from build123d import *

# Parameters (mm, degrees)
SKETCH1_R           = 15
BOSS_EXTRUDE1_DEPTH = 3


with BuildPart() as part:
    # Sketch1 → Boss-Extrude1 (new body)
    with BuildSketch(Plane(origin=(0, 0, 0), x_dir=(1, 0, 0), z_dir=(0, 1, 0))):
        with Locations(Location((0, 0, 0), (0, 0, 270))):
            Circle(SKETCH1_R)
        with BuildLine():
            Line((-1.118033989, 1), (1.118033989, 1))
            ThreePointArc((1.118033989, 1), (0, -1.5), (-1.118033989, 1))
        make_face(mode=Mode.SUBTRACT)
        with BuildLine():
            Line((-12.557368355, -7.25), (-10.392304845, -6))
            ThreePointArc((-10.392304845, -6), (-9.192533317, -7.713451316), (-7.713451316, -9.192533317))
            Line((-7.713451316, -9.192533317), (-9.32042034, -11.107644425))
            ThreePointArc((-9.32042034, -11.107644425), (-11.107644425, -9.32042034), (-12.557368355, -7.25))
        make_face(mode=Mode.SUBTRACT)
        with BuildLine():
            Line((-4.959292078, -13.625543001), (-4.10424172, -11.276311449))
            ThreePointArc((-4.10424172, -11.276311449), (-2.083778132, -11.817693036), (0, -12))
            Line((0, -12), (0, -14.5))
            ThreePointArc((0, -14.5), (-2.517898576, -14.279712419), (-4.959292078, -13.625543001))
        make_face(mode=Mode.SUBTRACT)
        with BuildLine():
            Line((4.959292078, -13.625543001), (4.10424172, -11.276311449))
            ThreePointArc((4.10424172, -11.276311449), (6, -10.392304845), (7.713451316, -9.192533317))
            Line((7.713451316, -9.192533317), (9.32042034, -11.107644425))
            ThreePointArc((9.32042034, -11.107644425), (7.25, -12.557368355), (4.959292078, -13.625543001))
        make_face(mode=Mode.SUBTRACT)
        with BuildLine():
            Line((12.557368355, -7.25), (10.392304845, -6))
            ThreePointArc((10.392304845, -6), (11.276311449, -4.10424172), (11.817693036, -2.083778132))
            Line((11.817693036, -2.083778132), (14.279712419, -2.517898576))
            ThreePointArc((14.279712419, -2.517898576), (13.625543001, -4.959292078), (12.557368355, -7.25))
        make_face(mode=Mode.SUBTRACT)
        with BuildLine():
            Line((-14.279712419, 2.517898576), (-11.817693036, 2.083778132))
            ThreePointArc((-11.817693036, 2.083778132), (-12, 0), (-11.817693036, -2.083778132))
            Line((-11.817693036, -2.083778132), (-14.279712419, -2.517898576))
            ThreePointArc((-14.279712419, -2.517898576), (-14.5, 0), (-14.279712419, 2.517898576))
        make_face(mode=Mode.SUBTRACT)
        with BuildLine():
            Line((-9.32042034, 11.107644425), (-7.713451316, 9.192533317))
            ThreePointArc((-7.713451316, 9.192533317), (-9.192533317, 7.713451316), (-10.392304845, 6))
            Line((-10.392304845, 6), (-12.557368355, 7.25))
            ThreePointArc((-12.557368355, 7.25), (-11.107644425, 9.32042034), (-9.32042034, 11.107644425))
        make_face(mode=Mode.SUBTRACT)
        with BuildLine():
            Line((-4.10424172, 11.276311449), (-4.959292078, 13.625543001))
            ThreePointArc((-4.959292078, 13.625543001), (-2.517898576, 14.279712419), (0, 14.5))
            Line((0, 14.5), (0, 12))
            ThreePointArc((0, 12), (-2.083778132, 11.817693036), (-4.10424172, 11.276311449))
        make_face(mode=Mode.SUBTRACT)
        with BuildLine():
            ThreePointArc((11.817693036, 2.083778132), (11.276311449, 4.10424172), (10.392304845, 6))
            Line((10.392304845, 6), (12.557368355, 7.25))
            ThreePointArc((12.557368355, 7.25), (13.625543001, 4.959292078), (14.279712419, 2.517898576))
            Line((14.279712419, 2.517898576), (11.817693036, 2.083778132))
        make_face(mode=Mode.SUBTRACT)
        with BuildLine():
            Line((9.32042034, 11.107644425), (7.713451316, 9.192533317))
            ThreePointArc((7.713451316, 9.192533317), (6, 10.392304845), (4.10424172, 11.276311449))
            Line((4.10424172, 11.276311449), (4.959292078, 13.625543001))
            ThreePointArc((4.959292078, 13.625543001), (7.25, 12.557368355), (9.32042034, 11.107644425))
        make_face(mode=Mode.SUBTRACT)
    extrude(amount=BOSS_EXTRUDE1_DEPTH)


solid = part.part
The listing builds one solid part. Answer for the finished solid, in the listing's coordinates (mm). Coordinates: 2 decimals unless noted, no trailing zeros. Write each loop counter-clockwise with the first axis right and the second up, starting at its lowest first coordinate (ties: lowest second). Pieces come first, ordered by that corner, then holes. Notation, with made-up numbers: M -35.5,28 L 21.5,28 A22 cw 21.5,61 Z; hole C 12,-31.75 d7. An arc over 180 degrees is marked long. Put each result on its own line as item: value. Start each with the question number.
1. Consider line 1 (X direction, y = 1, z = 6.25); line 2 (Z direction, x = 5, y = 0.45); line 3 (Z direction, x = -2.75, y = 0.45). Determine where each line is inside the solid, lowest interval first. Write a range as from..to.
2. Flat-ended cylindrical pins translate along their axes: P1, Ø4, axis at x = -12, z = -7.5, coming from the -Y side; P2, Ø1, axis at y = 1.5, z = 7.5, coming from the -X side; P3, Ø1.2, axis at y = 1.5, z = 14, coming from the -X side; P4, Ø1.5, axis at y = 2.5, z = 6, coming from the +X side. Find the tip coordinate at first contact, or state that the pin passes through.
3. For a pull along X with two mould halves and no side action, classify faces 1 (the cylindrical face through (-9.17, 1.48, -7.74)), 2 (the flat face through (0, 0, 3)) as pulls with the +X half, pulls with the -X half, needs draft (parallel to the pull), parting line crosses it, or undercut.
4. A cutting plane is placed at D-D on x = -8.25. Write down the section's boundary in (y, z).
5. A cutting plane is placed at B-B on x = 0.5. Write down the section's boundary in (y, z).
6. A cutting plane is placed at C-C on z = -4.5. Write down the section's boundary in (x, y).
7. A cutting plane is placed at A-A on z = 0. Write down the section's boundary in (x, y).
Resolved:
1. line 1: x = -13.64..-10.83, -10.24..10.83, 13.08..13.64
1. line 2: z = -14.14..-13.61, -10.91..10.91, 13.61..14.14
1. line 3: z = -14.75..-14.24, -11.68..11.68, 14.24..14.75
2. P1: stops at y = 0
2. P2: stops at x = -13.27
2. P3: stops at x = -6.74
2. P4: stops at x = 14.05
3. face 1: undercut
3. face 2: needs draft
4. outline: M 0,-12.53 L 3,-12.53 L 3,-9.83 L 0,-9.83 Z; M 0,-8.71 L 3,-8.71 L 3,8.71 L 0,8.71 Z; M 0,9.83 L 3,9.83 L 3,12.53 L 0,12.53 Z
5. outline: M 0,-14.99 L 3,-14.99 L 3,-1 L 0,-1 Z; M 0,1.41 L 3,1.41 L 3,14.99 L 0,14.99 Z
6. outline: M -14.31,0 L 11.12,0 L 11.12,3 L -14.31,3 Z; M 13.78,0 L 14.31,0 L 14.31,3 L 13.78,3 Z
7. outline: M -15,0 L -14.5,0 L -14.5,3 L -15,3 Z; M -12,0 L -1.5,0 L -1.5,3 L -12,3 Z; M 1.5,0 L 15,0 L 15,3 L 1.5,3 Z
